```python
from build123d import *

# Parameters (mm, degrees)
F0_W     = 125.5502849817
F0_H     = 126.5566982329
F1_DEPTH = 45.466
F2_R     = 12.4740683963
F3_DEPTH = 4.064


# Not quite as in the source:
# - a fillet or chamfer that OpenCascade refuses, or shapes differently, is made with other operations: its cross-section is extruded or revolved along the edge and cut away or added


with BuildPart() as f1:
    # F0 (on Front) → F1 (new body)
    with BuildSketch(Plane.XZ):
        with Locations((3.0192434788, -2.1386351436)):
            Rectangle(F0_W, F0_H)
    extrude(amount=F1_DEPTH)

    # F2 (on face) → F3 (join)
    with BuildSketch(Plane.XY.offset(61.1397139728)):
        with Locations((-41.892029345, -17.1090569347)):
            Circle(F2_R)
    extrude(amount=F3_DEPTH)

    # F4: fillet of radius 5.08 on 1 edges, made by hand

    # F4_s1 → F4_t2 (revolve, cut)
    with BuildSketch(Plane.XZ.offset(17.1090569347)):
        with BuildLine():
            ThreePointArc((-29.4179609488, 61.1397139728), (-31.1824500034, 64.0586650526), (-34.3953241061, 65.2037139728))
            Line((-34.3953241061, 65.2037139728), (-29.4179609488, 65.2037139728))
            Line((-29.4179609488, 65.2037139728), (-29.4179609488, 61.1397139728))
        make_face()
    revolve(axis=Axis((-41.892029345, -17.1090569347, 65.2037139728), (0, 0, 1)), mode=Mode.SUBTRACT)


solid = f1.part
```
Read the model definition and answer for the solid it produces. Units are mm, in the model's axes. Coordinates: 2 decimals unless noted, no trailing zeros. Loops run counter-clockwise (first coordinate to the right, second up) from the corner with the lowest first, then second, coordinate; pieces in that order, holes last. Notation, with made-up numbers: (1, 77.25) - (59, 77.25) arc R16 ccw to (59, 91.25) - close; hole circle Ø4 at (46.5, 73). An arc over 180 degrees is marked (long way). Answer in a Markdown table with one row per item.
1. Given pin 1 (12 mm diameter, centred on x = -43, y = -34.5, fed in from +Z); pin 2 (10 mm diameter, centred on x = 24.5, z = -46, fed in from +Y); pin 3 (3 mm diameter, centred on x = -20, y = -12, fed in from +Z), each flat-ended and moving along its own axis, determine where each tip first touches the part or whether it passes through.
Conclusion:
| item | result |
|---|---|
| pin 1 | stops at z = 63.34 |
| pin 2 | stops at y = 0 |
| pin 3 | stops at z = 61.14 |
2. Determine the mould class of faces 1 (the face through (2, 0, -1)), 2 (the face through (-42, -17, 65.204)), 3 (the face through (2, -22, -65.417)) for opening direction Z: +Z half, -Z half, draft (parallel to the pull), parting line (faces both ways), or undercut.
Conclusion:
| item | result |
|---|---|
| face 1 | draft |
| face 2 | +Z half |
| face 3 | -Z half |
3. Find section A-A, the plane x = 57.5. Write down the section's boundary in (y, z).
Conclusion:
| item | result |
|---|---|
| outline | (-45.47, -65.42) - (0, -65.42) - (0, 61.14) - (-45.47, 61.14) - close |
4. Straight lines are drawn through the part: line 1 (Z direction, x = 24.5, y = -40); line 2 (Z direction, x = -32.5, y = -14.5). For each, find the intervals that lie inside material, in ascending order.
Conclusion:
| item | result |
|---|---|
| line 1 | z = -65.42 to 61.14 |
| line 2 | z = -65.42 to 64.68 |
